Part model, mm, in its own coordinate system. A direction names the side the tool comes from. Round coordinates to 2 decimals unless told otherwise and drop trailing zeros. Loops run counter-clockwise (first coordinate to the right, second up) from the corner with the lowest first, then second, coordinate; pieces in that order, holes last.
1) Drop flat-ended pins along their axis: P1, Ø8, axis at y = 11.5, z = 32.5, coming from the +X side; P2, Ø3, axis at x = -45, y = 36.5, coming from the -Z side; P3, Ø3, axis at x = 33.5, z = 31, coming from the +Y side; P4, Ø8, axis at x = -18.5, z = 43.5, coming from the -Y side. Give the stop position or say it passes through.
2) Band-saw the part on C-C, the plane z = 46. Write the cut outline in (x, y) (3 decimals), then the cut area to 3 significant figures.
3) 3-axis set-ups, long thin cutter, end or side, ignore diameter. For faces 1 (the cylindrical face through (7.571, -34.094, 36.713)), 2 (the cylindrical face through (-2.93, 48.34, 9.39)): which of +Z, -Z, +X, -X, +Y, -Y reach the whole face in a straight line?
4) Band-saw the part on D-D, the plane z = 14. Write the cut outline in (x, y) (3 decimals), then the cut area to 3 significant figures.
5) Probe line 1 (Y direction, x = 0, z = 13) (3 decimals); line 2 (Y direction, x = 0, z = 22); line 3 (Z direction, x = 1, y = 42.5). List the from-to ranges inside material, lowest first.
6) Mould opens along X. For faces 3 (the cylindrical face through (-1.377, -47.776, 9.392)), 4 (the flat face through (-29, -29, 19.05)), 5 (the cylindrical face through (15.1, -68.2, 8)) say: +X half, -X half, draft (parallel to the pull), parting line (faces both ways), or undercut.
7) Band-saw the part on A-A, the plane y = 0. Write the cut outline in (x, z) (3 decimals), then the cut area to 3 significant figures.
from build123d import *

# Parameters (mm, degrees)
D_GAGEMENT_22_D              = 12.7
R_P_TITION_CIRCULAIRE1_COUNT = 4
CONG_1_R                     = 3.175


with BuildPart() as part:
    # Esquisse1 → Base-Révolution (revolve)
    with BuildSketch(Plane(origin=(0, 0, 0), x_dir=(0, 0, -1), z_dir=(1, 0, 0)), mode=Mode.PRIVATE) as base_r_volution_sk:
        Polygon((0, 19.05), (0, 69.85), (-19.05, 69.85), (-19.05, 34.925), (-53.975, 34.925), (-53.975, 19.05), align=None)
    revolve(base_r_volution_sk.sketch.rotate(Axis((0, 0, 48.319469853), (0, 0, -1)), 270), axis=Axis((0, 0, 48.319469853), (0, 0, -1)))

    # Dégagement 22 (through all)
    with Locations(Plane.XY.offset(19.05)):
        with Locations((0, 53.975)):
            d_gagement_22 = Hole(D_GAGEMENT_22_D / 2)

    # Répétition circulaire1: Dégagement 22 ×4 about axis
    r_p_tition_circulaire1_axis = Axis((0, 0, 0), (0, 0, 1))
    for i in range(1, R_P_TITION_CIRCULAIRE1_COUNT):
        add(d_gagement_22.rotate(r_p_tition_circulaire1_axis, i * 360 / R_P_TITION_CIRCULAIRE1_COUNT), mode=Mode.SUBTRACT)

    # Congé1
    cong_1_edges = [part.edges().sort_by_distance(p)[0] for p in [
        (34.925, 0, 53.975),
        (34.925, 0, 19.05),
        (69.85, 0, 19.05),
    ]]
    fillet(cong_1_edges, radius=CONG_1_R)


solid = part.part
Reported:
1. P1: stops at x = 34.11
1. P2: stops at z = 0
1. P3: stops at y = 13.99
1. P4: stops at y = -31.77
2. outline: circle Ø69.85 at (0, 0); hole circle Ø38.1 at (0, 0)
2. area: 2,690 mm2
3. face 1: +Z
3. face 2: +Z, -Z
4. outline: circle Ø139.7 at (0, 0); hole circle Ø12.7 at (-53.975, 0); hole circle Ø38.1 at (0, 0); hole circle Ø12.7 at (0, -53.975); hole circle Ø12.7 at (0, 53.975); hole circle Ø12.7 at (53.975, 0)
4. area: 13,700 mm2
5. line 1: y = -69.85 to -60.325, -47.625 to -19.05, 19.05 to 47.625, 60.325 to 69.85
5. line 2: y = -34.93 to -19.05, 19.05 to 34.93
5. line 3: z = 0 to 19.05
6. face 3: undercut
6. face 4: draft
6. face 5: parting line
7. outline: (-69.85, 0) - (-60.325, 0) - (-60.325, 19.05) - (-66.675, 19.05) arc R3.175 ccw to (-69.85, 15.875) - close; (-47.625, 0) - (-19.05, 0) - (-19.05, 53.975) - (-31.75, 53.975) arc R3.175 ccw to (-34.925, 50.8) - (-34.925, 22.225) arc R3.175 cw to (-38.1, 19.05) - (-47.625, 19.05) - close; (19.05, 0) - (47.625, 0) - (47.625, 19.05) - (38.1, 19.05) arc R3.175 cw to (34.925, 22.225) - (34.925, 50.8) arc R3.175 ccw to (31.75, 53.975) - (19.05, 53.975) - close; (60.325, 0) - (69.85, 0) - (69.85, 15.875) arc R3.175 ccw to (66.675, 19.05) - (60.325, 19.05) - close
7. area: 2,560 mm2
